from build123d import *

# Parameters (mm, degrees)
ESTRUSIONE_ESTRUSIONE1_DEPTH = 1
SCHIZZO2_W                   = 71.6
SCHIZZO2_H                   = 70
ESTRUSIONE_ESTRUSIONE2_DEPTH = 1
SCHIZZO3_R                   = 2
ESTRUSIONE_ESTRUSIONE3_DEPTH = 71.6


with BuildPart() as part:
    # Schizzo1 → Estrusione-Estrusione1 (new body)
    with BuildSketch(Plane(origin=(0, 0, 0), x_dir=(-1, 0, 0), z_dir=(0, 0, 1))):
        with BuildLine():
            Line((68, -41), (68, 74))
            Line((68, 74), (-75.894663844, 74))
            ThreePointArc((-75.894663844, 74), (-104.136158772, 19.790412733), (-97.749680306, -41))
            Line((-97.749680306, -41), (68, -41))
        make_face()
    extrude(amount=ESTRUSIONE_ESTRUSIONE1_DEPTH)

    # Schizzo2 → Estrusione-Estrusione2 (add)
    with BuildSketch(Plane(origin=(0, 0, 0), x_dir=(-1, 0, 0), z_dir=(0, 0, -1))):
        with Locations((-0.004840153, 76)):
            Rectangle(SCHIZZO2_W, SCHIZZO2_H)
    extrude(amount=-ESTRUSIONE_ESTRUSIONE2_DEPTH)

    # Schizzo3 → Estrusione-Estrusione3 (add)
    with BuildSketch(Plane.ZY.offset(35.795159847)):
        with BuildLine():
            Line((-61, 113.35913787), (0, 111))
            Line((0, 111), (0, 102.42172426))
            Line((0, 102.42172426), (-61, 104.78086213))
            ThreePointArc((-61, 104.78086213), (-65.28913787, 109.07), (-61, 113.35913787))
        make_face()
        with Locations((-61, 109.07)):
            Circle(SCHIZZO3_R, mode=Mode.SUBTRACT)
    extrude(amount=-ESTRUSIONE_ESTRUSIONE3_DEPTH)


solid = part.part
Read the model definition and answer for the solid it produces. Units are mm, in the model's axes. A direction names the side the tool comes from. Coordinates: 2 decimals unless noted, no trailing zeros. Order: outer loops, then holes, each group sorted by start corner. A loop starts at its lowest first (then second) coordinate and runs counter-clockwise, first axis right, second up. Notation, with made-up numbers: (22.5, 71.5) -> (37.5, 71.5) arc R21 cw to (37.5, 90.5) -> close; hole circle Ø8 at (16.5, 3.25). An arc over 180 degrees is marked (long way). Answer as a JSON object with one key per item and string values.
1) A tool of negligible diameter and unlimited length cuts with its end or side. For faces 4 (the face through (20, -7, 0)), 5 (the face through (20, -3, 1)), from which of +Z, -Z, +X, -X, +Y, -Y can it reach the whole face along a straight path? Write none if from no direction.
Model answer:
{"face 4": "-Z, +X, -X, -Y", "face 5": "+Z, +X, -X, +Y, -Y"}
2) A cutting plane is placed at A-A, the plane x = -8. Determine the outline of the cut face in (y, z), plus the area to 3 significant figures.
Model answer:
{"outline": "(-74, 0) -> (102.42, 0) -> (104.78, -61) arc R4.29 ccw to (113.36, -61) -> (111, 0) -> (111, 1) -> (-74, 1) -> close; hole circle Ø4 at (109.07, -61)", "area": "725 mm²"}
3) Consider line 1 along Y through (x, z) = (-18, -61); line 2 along Z through (x, y) = (10, -34.5); line 3 along Z through (x, y) = (-5, 109). Determine where each line is inside the solid, lowest interval first. Write a range as from..to.
Model answer:
{"line 1": "y = 104.78..107.07, 111.07..113.36", "line 2": "z = 0..1", "line 3": "z = -65.29..-63, -59..1"}
4) A cutting plane is placed at C-C, the plane z = -40. Determine the outline of the cut face in (x, y), plus the area to 3 significant figures.
Model answer:
{"outline": "(-35.8, 103.97) -> (35.8, 103.97) -> (35.8, 112.55) -> (-35.8, 112.55) -> close", "area": "614 mm²"}
5) Each of these flat-tipped pins is pushed along its axis until it touches: pin 1 (8 mm diameter, centred on x = -6.5, y = 74.5, fed in from -Z); pin 2 (8 mm diameter, centred on x = -12.5, z = -45.5, fed in from +Y); pin 3 (0.5 mm diameter, centred on x = 70, z = 0.5, fed in from +Y). Where does it stop, or does it pass through?
Model answer:
{"pin 1": "stops at z = 0", "pin 2": "stops at y = 112.91", "pin 3": "stops at y = 41"}
6) The mould has two halves that part along Z. Classify faces 1 (the face through (35.805, 107, -32)), 2 (the face through (-0.496, 111.053, -61.26)), 3 (the face through (-0.496, 112.196, -30.927)): released by +Z, released by -Z, zero draft, split by the parting line, or undercut.
Model answer:
{"face 1": "zero draft", "face 2": "undercut", "face 3": "released by +Z"}
7) A cutting plane is placed at B-B, the plane y = -57.5. Determine the outline of the cut face in (x, z), plus the area to 3 significant figures.
Model answer:
{"outline": "(-68, 0) -> (89.05, 0) -> (89.05, 1) -> (-68, 1) -> close", "area": "157 mm²"}
